CAD build for the part. Positions are in the model's coordinates, mm. Give positions to 0.01 mm unless a question says otherwise; leave off trailing zeros. Loops run counter-clockwise (first coordinate to the right, second up) from the corner with the lowest first, then second, coordinate; pieces in that order, holes last. Notation, with made-up numbers: (-29, 30.25) - (14, 30.25) arc R20 ccw to (14, 54.25) - close; hole circle Ø3 at (88.25, -34.75). An arc over 180 degrees is marked (long way). Return JSON: item names as keys, results as strings.
from build123d import *

# Parameters (mm, degrees)
F0_R     = 4.38125
F0_R_2   = 2.38125
F1_DEPTH = 20
F2_R     = 2.38125
F3_DEPTH = 5


with BuildPart() as f1:
    # F0 (on Top) → F1 (new body)
    with BuildSketch(Plane.XY):
        Circle(F0_R)
        Circle(F0_R_2, mode=Mode.SUBTRACT)
    extrude(amount=F1_DEPTH)

    # F2 (on face) → F3 (join)
    with BuildSketch(Plane(origin=(0, 0, 0), x_dir=(1, 0, 0), z_dir=(0, 0, -1))):
        with BuildLine():
            Line((-4.38125, 15), (-4.38125, 0))
            ThreePointArc((-4.38125, 0), (0, -4.38125), (4.38125, 0))
            Line((4.38125, 0), (4.38125, 15))
            ThreePointArc((4.38125, 15), (0, 19.38125), (-4.38125, 15))
        make_face()
        Circle(F2_R, mode=Mode.SUBTRACT)
    extrude(amount=F3_DEPTH)


solid = f1.part
1. Cut at C-C, the plane z = 11.5. Write the cut outline in (x, y).
Values follow:
{"outline": "circle Ø8.76 at (0, 0); hole circle Ø4.76 at (0, 0)"}
2. Cut at A-A, the plane x = 0. Write the cut outline in (y, z), plus the area to 3 significant figures.
Values follow:
{"outline": "(-19.38, -5) - (-2.38, -5) - (-2.38, 20) - (-4.38, 20) - (-4.38, 0) - (-19.38, 0) - close; (2.38, -5) - (4.38, -5) - (4.38, 20) - (2.38, 20) - close", "area": "175 mm²"}
3. Cut at D-D, the plane y = -12. Write the cut outline in (x, z).
Values follow:
{"outline": "(-4.38, -5) - (4.38, -5) - (4.38, 0) - (-4.38, 0) - close"}
4. Cut at B-B, the plane y = 1.25. Write the cut outline in (x, z).
Values follow:
{"outline": "(-4.2, -5) - (-2.03, -5) - (-2.03, 20) - (-4.2, 20) - close; (2.03, -5) - (4.2, -5) - (4.2, 20) - (2.03, 20) - close"}
5. Drill centre lines: probe 1 along Y at (x, z) = (0, -3.2); probe 2 along Y at (x, z) = (0, 9.75); probe 3 along Z at (x, y) = (-2.25, -15.25). Where is each one in solid material? Low to high.
Values follow:
{"probe 1": "y = -19.38 to -2.38, 2.38 to 4.38", "probe 2": "y = -4.38 to -2.38, 2.38 to 4.38", "probe 3": "z = -5 to 0"}
6. Drop flat-ended pins along their axis: P1, Ø2, axis at x = 2, z = 6.5, coming from the +Y side; P2, Ø4, axis at x = 0, y = 0, coming from the +Z side; P3, Ø4, axis at x = 0.5, z = 13.5, coming from the -Y side. Give the stop position or say it passes through.
Values follow:
{"P1": "stops at y = 4.27", "P2": "passes through", "P3": "stops at y = -4.38"}
